```python
from build123d import *

# Parameters (mm, degrees)
SKETCH1_W           = 52
SKETCH1_H           = 92
BOSS_EXTRUDE1_DEPTH = 10
SKETCH2_W           = 10
SKETCH2_H           = 52
BOSS_EXTRUDE2_DEPTH = 20
CUT_EXTRUDE1_REACH  = 109.555
SKETCH3_R           = 3
SKETCH3_R_2         = 5
SKETCH3_R_3         = 2.5
CUT_EXTRUDE2_REACH  = 107.489
SKETCH4_R           = 3


with BuildPart() as part:
    # Sketch1 → Boss-Extrude1 (new body)
    with BuildSketch(Plane(origin=(0, 0, 0), x_dir=(1, 0, 0), z_dir=(0, 1, 0))):
        with Locations((26, 46)):
            Rectangle(SKETCH1_W, SKETCH1_H)
    extrude(amount=BOSS_EXTRUDE1_DEPTH)

    # Sketch2 → Boss-Extrude2 (add)
    with BuildSketch(Plane(origin=(0, 10, 0), x_dir=(1, 0, 0), z_dir=(0, 1, 0))):
        with Locations((5, 66)):
            Rectangle(SKETCH2_W, SKETCH2_H)
    extrude(amount=BOSS_EXTRUDE2_DEPTH)

    # Sketch3 → Cut-Extrude1 (cut, up to next)
    with BuildSketch(Plane(origin=(0, 10, 0), x_dir=(1, 0, 0), z_dir=(0, 1, 0)), mode=Mode.PRIVATE) as cut_extrude1_sk1:
        with Locations(Location((42, 30, 0), (0, 0, 270))):
            Circle(SKETCH3_R)
    cut_extrude1_tool1 = extrude(cut_extrude1_sk1.sketch, amount=-CUT_EXTRUDE1_REACH, mode=Mode.PRIVATE) & part.part
    # Sketch3 → Cut-Extrude1 (cut, up to next)
    with BuildSketch(Plane(origin=(0, 10, 0), x_dir=(1, 0, 0), z_dir=(0, 1, 0)), mode=Mode.PRIVATE) as cut_extrude1_sk2:
        with Locations(Location((10, 30, 0), (0, 0, 270))):
            Circle(SKETCH3_R)
    cut_extrude1_tool2 = extrude(cut_extrude1_sk2.sketch, amount=-CUT_EXTRUDE1_REACH, mode=Mode.PRIVATE) & part.part
    # Sketch3 → Cut-Extrude1 (cut, up to next)
    with BuildSketch(Plane(origin=(0, 10, 0), x_dir=(1, 0, 0), z_dir=(0, 1, 0)), mode=Mode.PRIVATE) as cut_extrude1_sk3:
        with Locations(Location((42, 10, 0), (0, 0, 270))):
            Circle(SKETCH3_R)
    cut_extrude1_tool3 = extrude(cut_extrude1_sk3.sketch, amount=-CUT_EXTRUDE1_REACH, mode=Mode.PRIVATE) & part.part
    # Sketch3 → Cut-Extrude1 (cut, up to next)
    with BuildSketch(Plane(origin=(0, 10, 0), x_dir=(1, 0, 0), z_dir=(0, 1, 0)), mode=Mode.PRIVATE) as cut_extrude1_sk4:
        with Locations(Location((10, 10, 0), (0, 0, 270))):
            Circle(SKETCH3_R)
    cut_extrude1_tool4 = extrude(cut_extrude1_sk4.sketch, amount=-CUT_EXTRUDE1_REACH, mode=Mode.PRIVATE) & part.part
    # Sketch3 → Cut-Extrude1 (cut, up to next)
    with BuildSketch(Plane(origin=(0, 10, 0), x_dir=(1, 0, 0), z_dir=(0, 1, 0)), mode=Mode.PRIVATE) as cut_extrude1_sk5:
        with Locations(Location((28.45, 68.45, 0), (0, 0, 270))):
            Circle(SKETCH3_R_2)
    cut_extrude1_tool5 = extrude(cut_extrude1_sk5.sketch, amount=-CUT_EXTRUDE1_REACH, mode=Mode.PRIVATE) & part.part
    # Sketch3 → Cut-Extrude1 (cut, up to next)
    with BuildSketch(Plane(origin=(0, 10, 0), x_dir=(1, 0, 0), z_dir=(0, 1, 0)), mode=Mode.PRIVATE) as cut_extrude1_sk6:
        with Locations(Location((41.354698757, 81.354698757, 0), (0, 0, 270))):
            Circle(SKETCH3_R_3)
    cut_extrude1_tool6 = extrude(cut_extrude1_sk6.sketch, amount=-CUT_EXTRUDE1_REACH, mode=Mode.PRIVATE) & part.part
    # Sketch3 → Cut-Extrude1 (cut, up to next)
    with BuildSketch(Plane(origin=(0, 10, 0), x_dir=(1, 0, 0), z_dir=(0, 1, 0)), mode=Mode.PRIVATE) as cut_extrude1_sk7:
        with Locations(Location((15.545301243, 55.545301243, 0), (0, 0, 270))):
            Circle(SKETCH3_R_3)
    cut_extrude1_tool7 = extrude(cut_extrude1_sk7.sketch, amount=-CUT_EXTRUDE1_REACH, mode=Mode.PRIVATE) & part.part
    add(cut_extrude1_tool1.solids().sort_by_distance((42, 10, -30))[0], mode=Mode.SUBTRACT)
    add(cut_extrude1_tool2.solids().sort_by_distance((10, 10, -30))[0], mode=Mode.SUBTRACT)
    add(cut_extrude1_tool3.solids().sort_by_distance((42, 10, -10))[0], mode=Mode.SUBTRACT)
    add(cut_extrude1_tool4.solids().sort_by_distance((10, 10, -10))[0], mode=Mode.SUBTRACT)
    add(cut_extrude1_tool5.solids().sort_by_distance((28.45, 10, -68.45))[0], mode=Mode.SUBTRACT)
    add(cut_extrude1_tool6.solids().sort_by_distance((41.354699, 10, -81.354699))[0], mode=Mode.SUBTRACT)
    add(cut_extrude1_tool7.solids().sort_by_distance((15.545301, 10, -55.545301))[0], mode=Mode.SUBTRACT)

    # Sketch4 → Cut-Extrude2 (cut, up to next)
    with BuildSketch(Plane(origin=(10, 0, 0), x_dir=(0, 0, -1), z_dir=(1, 0, 0)), mode=Mode.PRIVATE) as cut_extrude2_sk1:
        with Locations((50, 20.005)):
            Circle(SKETCH4_R)
    cut_extrude2_tool1 = extrude(cut_extrude2_sk1.sketch, amount=-CUT_EXTRUDE2_REACH, mode=Mode.PRIVATE) & part.part
    # Sketch4 → Cut-Extrude2 (cut, up to next)
    with BuildSketch(Plane(origin=(10, 0, 0), x_dir=(0, 0, -1), z_dir=(1, 0, 0)), mode=Mode.PRIVATE) as cut_extrude2_sk2:
        with Locations((82, 20.005)):
            Circle(SKETCH4_R)
    cut_extrude2_tool2 = extrude(cut_extrude2_sk2.sketch, amount=-CUT_EXTRUDE2_REACH, mode=Mode.PRIVATE) & part.part
    add(cut_extrude2_tool1.solids().sort_by_distance((10, 20.005, -50))[0], mode=Mode.SUBTRACT)
    add(cut_extrude2_tool2.solids().sort_by_distance((10, 20.005, -82))[0], mode=Mode.SUBTRACT)


solid = part.part
```
CAD build for the part. Positions are in the model's coordinates, mm. A direction names the side the tool comes from. Round coordinates to 2 decimals unless told otherwise and drop trailing zeros. Order: outer loops, then holes, each group sorted by start corner. A loop starts at its lowest first (then second) coordinate and runs counter-clockwise, first axis right, second up. Notation, with made-up numbers: (20, -12) -> (56, -12) arc R21 ccw to (56, -4) -> close; hole circle Ø5 at (-27.5, 8). An arc over 180 degrees is marked (long way). One line per question, with ' | ' between items.
Q1. Two-plate mould, pull along X, no slides. Class faces 1 (the flat face through (0, 11, -56)), 2 (the flat face through (10, 20, -66)), 3 (the flat face through (26, 5, 0)), 4 (the cylindrical face through (39.137, 5.07, -80.201)): released by +X, released by -X, zero draft, split by the parting line, or undercut.
Completed:
face 1: released by -X | face 2: released by +X | face 3: zero draft | face 4: undercut
Q2. Which spindle directions (+Z, -Z, +X, -X, +Y, -Y) get a long thin tool onto all of the face, cutting with end or side? Do faces 5 (the flat face through (5, 20, -40)), 6 (the cylindrical face through (10, 5, -13)). Say none if no direction does.
Completed:
face 5: +Z, +X, -X, +Y | face 6: +Y, -Y
Q3. Drop flat-ended pins along their axis: pin 1 (5.5 mm diameter, centred on y = 20.005, z = -50, fed in from +X); pin 2 (10 mm diameter, centred on y = 26.5, z = -57.5, fed in from +X); pin 3 (10 mm diameter, centred on x = 28, z = -24.5, fed in from -Y); pin 4 (8 mm diameter, centred on x = 41.35, z = -81.35, fed in from +Y). Give the stop position or say it passes through.
Completed:
pin 1: passes through | pin 2: stops at x = 10 | pin 3: stops at y = 0 | pin 4: stops at y = 10
Q4. Probe probe 1 along X at (y, z) = (6.5, -30); probe 2 along Y at (x, z) = (13, -77.5). List the from-to ranges inside material, lowest first.
Completed:
probe 1: x = 0 to 7, 13 to 39, 45 to 52 | probe 2: y = 0 to 10
Q5. Slice it at B-B (z = -50). Write the cut outline in (x, y) (3 decimals).
Completed:
outline: (0, 0) -> (52, 0) -> (52, 10) -> (10, 10) -> (10, 17.005) -> (0, 17.005) -> close; (0, 23.005) -> (10, 23.005) -> (10, 30) -> (0, 30) -> close
Q6. Slice it at A-A (x = 28.45). Write the cut outline in (y, z).
Completed:
outline: (0, -92) -> (10, -92) -> (10, -73.45) -> (0, -73.45) -> close; (0, -63.45) -> (10, -63.45) -> (10, 0) -> (0, 0) -> close
Q7. Slice it at D-D (x = 9). Write the cut outline in (y, z) (3 decimals).
Completed:
outline: (0, -92) -> (30, -92) -> (30, -40) -> (10, -40) -> (10, -32.828) -> (0, -32.828) -> close; (0, -27.172) -> (10, -27.172) -> (10, -12.828) -> (0, -12.828) -> close; (0, -7.172) -> (10, -7.172) -> (10, 0) -> (0, 0) -> close; hole circle Ø6 at (20.005, -82); hole circle Ø6 at (20.005, -50)
Q8. Slice it at C-C (z = -30). Write the cut outline in (x, y).
Completed:
outline: (0, 0) -> (7, 0) -> (7, 10) -> (0, 10) -> close; (13, 0) -> (39, 0) -> (39, 10) -> (13, 10) -> close; (45, 0) -> (52, 0) -> (52, 10) -> (45, 10) -> close
